Design review of the part shown in the three views and the two pictorial views. Dimensions are in mm from the part's minimum x, y and z. Round coordinates to 2 decimals unless told otherwise and drop trailing zeros. Order: outer loops, then holes, each group sorted by start corner. A loop starts at its lowest first (then second) coordinate and runs counter-clockwise, first axis right, second up. Notation, with made-up numbers: M 58.25,-22.75 L 67.25,-22.75 A13 cw 67.25,0.25 Z; hole C -10,81.5 d5. An arc over 180 degrees is marked long. Use a Markdown table: item, result. Add a question column.
(1) Take a section at C-C (x = 27). Write out the cut boundary in (y, z).
(2) The part is to be moulded in two halves that separate along X. For the marked faces 1 and 2, say which applies: released by +X, released by -X, zero draft, split by the parting line, or undercut.
(3) Take a section at D-D (z = 23). Write out the cut boundary in (x, y).
(4) For pin 1 (2 mm diameter, centred on x = 26, y = 16, fed in from -Z); pin 2 (2.5 mm diameter, centred on x = 18.5, z = 14, fed in from +Y); pin 3 (8 mm diameter, centred on x = 27, z = 4.5, fed in from +Y); pin 4 (4 mm diameter, centred on x = 4, z = 12.5, fed in from -Y), all flat-tipped, find the tip position at first contact; note any pin that passes through.
(5) Take a section at A-A (z = 12). Write out the cut boundary in (x, y).
(6) Take a section at B-B (y = 8.5). Write out the cut boundary in (x, z).
(7) To check wall thickness, follow probe 1 along Y at (x, z) = (8.95, 23); probe 2 along Z at (x, y) = (5, 15.6); probe 3 along X at (y, z) = (5.25, 14.5). State the ranges of each line that lie inside material, in increasing order. Write a range as from..to.
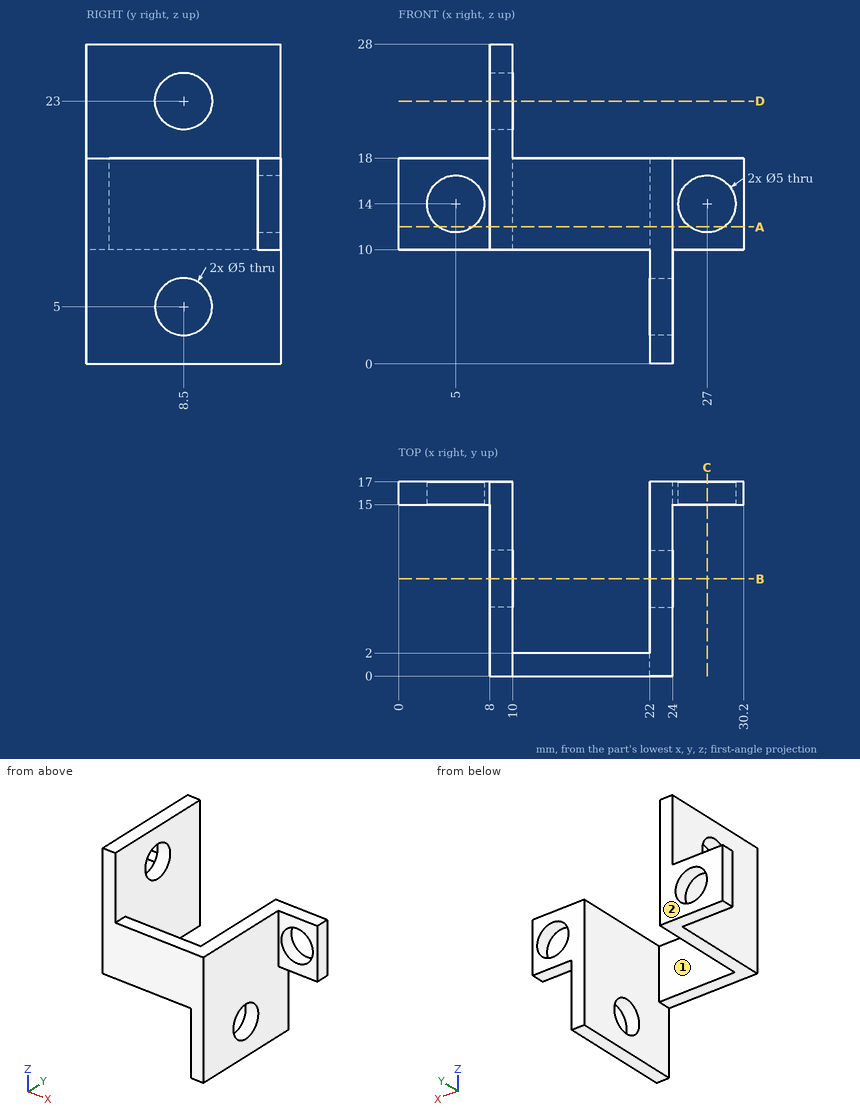
Verdict:
| question | item | result |
|---|---|---|
| 1 | outline | M 15,10 L 17,10 L 17,11.5 L 15,11.5 Z; M 15,16.5 L 17,16.5 L 17,18 L 15,18 Z |
| 2 | face 1 | undercut |
| 2 | face 2 | zero draft |
| 3 | outline | M 8,0 L 10,0 L 10,6 L 8,6 Z; M 8,11 L 10,11 L 10,17 L 8,17 Z |
| 4 | pin 1 | stops at z = 10 |
| 4 | pin 2 | stops at y = 2 |
| 4 | pin 3 | stops at y = 17 |
| 4 | pin 4 | stops at y = 15 |
| 5 | outline | M 0,15 L 3.5,15 L 3.5,17 L 0,17 Z; M 6.5,15 L 8,15 L 8,0 L 24,0 L 24,15 L 25.5,15 L 25.5,17 L 22,17 L 22,2 L 10,2 L 10,17 L 6.5,17 Z; M 28.5,15 L 30.2,15 L 30.2,17 L 28.5,17 Z |
| 6 | outline | M 8,10 L 10,10 L 10,20.5 L 8,20.5 Z; M 8,25.5 L 10,25.5 L 10,28 L 8,28 Z; M 22,0 L 24,0 L 24,2.5 L 22,2.5 Z; M 22,7.5 L 24,7.5 L 24,18 L 22,18 Z |
| 7 | probe 1 | y = 0..6, 11..17 |
| 7 | probe 2 | z = 10..11.5, 16.5..18 |
| 7 | probe 3 | x = 8..10, 22..24 |
